For this review, take the finished solid that the model builds, in its own axes (mm). A direction names the side the tool comes from. Coordinates: 2 decimals unless noted, no trailing zeros. Write each loop counter-clockwise with the first axis right and the second up, starting at its lowest first coordinate (ties: lowest second). Pieces come first, ordered by that corner, then holes. Notation, with made-up numbers: M 41.25,-3.5 L 84.25,-3.5 A21 ccw 84.25,1.5 Z; hole C 20,-31 d9. An arc over 180 degrees is marked long. Return JSON: item names as keys, results as strings.
Autodesk Inventor part; units mm, degrees
ref_plane "Start Plane" through (0, 0, 0) normal (0, 0, 1) x (1, 0, 0)
ref_plane "End Plane" through (0, 0, 39) normal (0, 0, 1) x (1, 0, 0)
ref_plane "YZ Plane" through (0, 0, 0) normal (1, 0, 0) x (0, 1, 0)
ref_plane "Start Plane" through (0, 0, 0) normal (0, 0, 1) x (1, 0, 0)
ref_plane "End Plane" through (0, 0, 39) normal (0, 0, 1) x (1, 0, 0)
sketch "Sketch" plane through (0, 0, 0) normal (0, 0, 1) x (1, 0, 0)
  circle A0 centre (0, 0) radius 11
  dimension "d0" = 22
extrude "Body" add sketch "Sketch" along normal up to surface (39 mm away) from surface at 0
sketch "Sketch3" plane through (0, 0, 0) normal (0, 0, 1) x (1, 0, 0)
  line L0 (0, 0) -> (10, 0)
ref_plane "Work Plane3" through (0, 0, 0) normal (0, -1, 0) x (1, 0, 0)
sketch "Sketch4" plane through (0, 0, 0) normal (0, -1, 0) x (1, 0, 0)
  line L0 (-2, 0) -> (12, 0)
  line L1 (-2, 39) -> (12, 39)
  dimension "d8" = 39
sketch "Sketch5" plane through (0, 0, 39) normal (0, 0, 1) x (1, 0, 0)
  circle A0 centre (0, 0) radius 7.5
  circle A1 centre (0, 0) radius 10.7703
  dimension "d9" = 15
extrude "Extrusion2" add sketch "Sketch5" along normal blind 17.5 contours A0
sketch "Sketch6" plane through (0, 0, 39) normal (0, 0, 1) x (1, 0, 0)
  circle A0 centre (0, 0) radius 11
  circle A1 centre (0, 0) radius 7.5
extrude "Extrusion3" cut sketch "Sketch6" against normal blind 1.5
sketch "Sketch7" plane through (0, 0, 0) normal (0, 0, -1) x (-1, 0, 0)
  circle A0 centre (0, 0) radius 7.5
  dimension "d16" = 15
extrude "Extrusion4" add sketch "Sketch7" along normal blind 17.5
sketch "Sketch8" plane through (0, 0, 0) normal (0, 0, -1) x (-1, 0, 0)
  circle A0 centre (0, 0) radius 7.5
  circle A1 centre (0, 0) radius 11
extrude "Extrusion5" cut sketch "Sketch8" against normal blind 1.5
equation "\"d0\" = G_H"
equation "\"d1\" = G_L"
equation "\"d16\" = d9"
equation "\"G_H\" = 22"
equation "\"G_L\" = d8"
equation "\"G_OFFSET_START\" = 0"
equation "\"G_OFFSET_END\" = 0"
equation "\"d5\" = G_OFFSET_END + B_L"
equation "\"B_L\" = 39"
equation "\"G_D\" = 22"
properties part number "ISO 1035/1 - 22 - 39" material "Steel, Mild"
1. We need section A-A (y = 0). State the section outline as (x, z) points, plus the area to 3 significant figures.
Checks:
{"outline": "M -11,1.5 L -7.5,1.5 L -7.5,-17.5 L 7.5,-17.5 L 7.5,1.5 L 11,1.5 L 11,37.5 L 7.5,37.5 L 7.5,56.5 L -7.5,56.5 L -7.5,37.5 L -11,37.5 Z", "area": "1,360 mm2"}
2. Clearance check with flat-ended pins moving along their axes: pin 1 Ø2 at (y, z) = (-2, -4) entering from +X; pin 2 Ø1 at (x, z) = (-1, -7) entering from +Y; pin 3 Ø2 at (y, z) = (-4, 17.5) entering from -X. State where each tip first meets the part, or that it passes through.
Checks:
{"pin 1": "x = 7.43", "pin 2": "y = 7.48", "pin 3": "x = -10.58"}
3. Wall thickness on L1, parallel to Z at x = 8.5, y = 0.75; L2, parallel to X at y = 1, z = -12; L3, parallel to X at y = 3.75, z = -1.5: over which ranges is each line inside the solid? List them lowest first. Write a range as from..to.
Checks:
{"L1": "1.5..37.5", "L2": "-7.43..7.43", "L3": "-6.5..6.5"}
4. For faces 1 (the face through (-7.2, 2.6, 1.5)), 2 (the face through (7.2, 2.6, 37.5)), 3 (the face through (0, 0, -17.5)), list the 3-axis set-ups (+Z, -Z, +X, -X, +Y, -Y) from which the entire face can be reached by the end or side of a thin tool; tool diameter is ignored.
Checks:
{"face 1": "-Z", "face 2": "+Z", "face 3": "-Z, +X, -X, +Y, -Y"}
5. We need section C-C (z = 49). State the section outline as (x, y) points, plus the area to 3 significant figures.
Checks:
{"outline": "C 0,0 d15", "area": "177 mm2"}
6. We need section D-D (z = 17). State the section outline as (x, y) points, plus the area to 3 significant figures.
Checks:
{"outline": "C 0,0 d22", "area": "380 mm2"}
